Geometry: final body of the model. Coordinates: model frame, mm. A direction names the side the tool comes from. Round coordinates to 2 decimals unless told otherwise and drop trailing zeros. Loops run counter-clockwise (first coordinate to the right, second up) from the corner with the lowest first, then second, coordinate; pieces in that order, holes last. Notation, with made-up numbers: (69.25, 78.5) - (85.25, 78.5) arc R26 cw to (85.25, 114.5) - close; hole circle Ø6 at (-7.75, 65). An arc over 180 degrees is marked (long way). Answer as a JSON object with one key per item and string values. Group by question number.
Item 1: First-contact query: pin 1 (2 mm diameter, centred on x = 21.5, y = 7.5, fed in from -Z); pin 2 (12 mm diameter, centred on y = 9, z = 40.5, fed in from +X) (3 decimals); pin 3 (8 mm diameter, centred on x = 23, y = 17, fed in from +Z); pin 4 (1.5 mm diameter, centred on x = 15.5, z = 23.5, fed in from +Y). Flat tips, straight axial feed; report the tip coordinate or a pass-through.
Item 2: Section C-C (z = 69.5). Return the cut outline in (x, y) (1 decimal), plus the area to 3 significant figures.
Item 3: Reachability of faces 1 (the face through (14, 17.064, 1)), 2 (the face through (4, 12, 1)), 3 (the face through (14.241, 16.004, 31.594)), 4 (the face through (20.63, 9.49, 68.44)), 5 (the face through (20.57, 8.45, 1.48)) from +Z, -Z, +X, -X, +Y, -Y: full face, straight path, thin tool, end or side. Return the list, or none.
Item 4: Line query: line 1 (Z direction, x = 27, y = 25.25); line 2 (Z direction, x = 18.75, y = 10.75); line 3 (Z direction, x = 13, y = 7.25). Output: solid intervals per line, ascending.
Item 5: Section B-B (z = 12.5). Return the cut outline in (x, y) (1 decimal).
Item 6: Section A-A (y = 2.25). Return the cut outline in (x, z).
Item 7: Draft query along Z for faces 6 (the face through (22, 14, 1)), 7 (the face through (14.3, 17.3, 3)). Return one class per face: released by +Z, released by -Z, zero draft, split by the parting line, or undercut.
Autodesk Fusion 360 part; units mm, degrees
sketch "Sketch1" plane through (0, 0, 0) normal (0, 0, 1) x (1, 0, 0)
  line L0 (29, 1.5) -> (29, 26.5)
  line L1 (27.5, 28) -> (1.5, 28)
  line L2 (0, 26.5) -> (0, 1.5)
  line L3 (3, 0) -> (3, 23.5595)
  line L4 (4.5, 25.0595) -> (24.5, 25.0595)
  line L5 (26, 23.5595) -> (26, 4.5)
  line L6 (24.5, 3) -> (8.5, 3)
  line L7 (4, 3) -> (4, 1.5)
  line L8 (4, 3) -> (4, 22.4878)
  line L9 (5.5, 23.9878) -> (23.5, 23.9878)
  line L10 (25, 22.4878) -> (25, 5.5)
  line L11 (23.5, 4) -> (9.5, 4)
  line L12 (8, 5.5) -> (8, 18.4723)
  line L13 (9.5, 19.9723) -> (19.5, 19.9723)
  line L14 (21, 18.4723) -> (21, 9.5)
  line L15 (19.5, 8) -> (13.5173, 8)
  line L16 (12.0173, 9.5) -> (12.0173, 14.3549)
  line L17 (14.0173, 16.3549) -> (15.0961, 16.3549)
  line L18 (17.0961, 14.3549) -> (17.0961, 11)
  line L19 (7, 4.5) -> (7, 19.6029)
  line L20 (8.5, 21.1029) -> (20.5, 21.1029)
  line L21 (22, 19.6029) -> (22, 8.5)
  line L22 (20.5, 7) -> (12.5, 7)
  line L23 (11, 8.5) -> (11, 15.5643)
  line L24 (12.5, 17.0643) -> (16.5, 17.0643)
  line L25 (18, 15.5643) -> (18, 12.3765)
  line L26 (1.5, 0) -> (3, 0)
  line L27 (5.5, 0) -> (27.5, 0)
  circle A0 centre (14.675, 14.0515) radius 2
  arc A1 (1.5, 28) -> (0, 26.5) centre (1.5, 26.5) ccw
  arc A2 (0, 1.5) -> (1.5, 0) centre (1.5, 1.5) ccw
  arc A3 (4.5, 25.0595) -> (3, 23.5595) centre (4.5, 23.5595) ccw
  arc A4 (26, 23.5595) -> (24.5, 25.0595) centre (24.5, 23.5595) ccw
  arc A5 (29, 26.5) -> (27.5, 28) centre (27.5, 26.5) ccw
  arc A6 (27.5, 0) -> (29, 1.5) centre (27.5, 1.5) ccw
  arc A7 (4, 1.5) -> (5.5, 0) centre (5.5, 1.5) ccw
  arc A8 (5.5, 23.9878) -> (4, 22.4878) centre (5.5, 22.4878) ccw
  arc A9 (25, 22.4878) -> (23.5, 23.9878) centre (23.5, 22.4878) ccw
  arc A10 (23.5, 4) -> (25, 5.5) centre (23.5, 5.5) ccw
  arc A11 (24.5, 3) -> (26, 4.5) centre (24.5, 4.5) ccw
  arc A12 (7, 4.5) -> (8.5, 3) centre (8.5, 4.5) ccw
  arc A13 (8, 5.5) -> (9.5, 4) centre (9.5, 5.5) ccw
  arc A14 (9.5, 19.9723) -> (8, 18.4723) centre (9.5, 18.4723) ccw
  arc A15 (8.5, 21.1029) -> (7, 19.6029) centre (8.5, 19.6029) ccw
  arc A16 (22, 19.6029) -> (20.5, 21.1029) centre (20.5, 19.6029) ccw
  arc A17 (21, 18.4723) -> (19.5, 19.9723) centre (19.5, 18.4723) ccw
  arc A18 (20.5, 7) -> (22, 8.5) centre (20.5, 8.5) ccw
  arc A19 (19.5, 8) -> (21, 9.5) centre (19.5, 9.5) ccw
  arc A20 (11, 8.5) -> (12.5, 7) centre (12.5, 8.5) ccw
  arc A21 (12.5, 17.0643) -> (11, 15.5643) centre (12.5, 15.5643) ccw
  arc A22 (18, 15.5643) -> (16.5, 17.0643) centre (16.5, 15.5643) ccw
  arc A23 (17.0961, 11) -> (18, 12.3765) centre (16.5, 12.3765) ccw
  arc A24 (14.0173, 16.3549) -> (12.0173, 14.3549) centre (14.0173, 14.3549) ccw
  arc A25 (17.0961, 14.3549) -> (15.0961, 16.3549) centre (15.0961, 14.3549) ccw
  arc A26 (12.0173, 9.5) -> (13.5173, 8) centre (13.5173, 9.5) ccw
  point P0 (29, 0)
  point P1 (0, 28)
  dimension "d1" = 29
  dimension "d2" = 28
  dimension "d3" = 4
  dimension "d4" = 1.5
  dimension "d5" = 2
  dimension "d15" = 1.5
extrude "Extrude1" add sketch "Sketch1" along normal blind 3
extrude "Extrude2" add sketch "Sketch1" along normal blind 61 contours A0
sketch "Sketch2" plane through (0, 0, 61) normal (0, 0, 1) x (-1, 0, 0)
  circle A0 centre (-14.675, -14.0515) radius 2
  circle A1 centre (-14.675, -14.0515) radius 7.5
  dimension "d10" = 15
extrude "Extrude3" add sketch "Sketch2" along normal blind 15 contours A0 | A1
fillet "Fillet1" radius 3 2 edges at (21.6674, 16.7636, 76) (21.6674, 16.7636, 61)
equation "d8 = 36 mm + 25 mm"
Values:
{
 "1": {"pin 1": "stops at z = 0", "pin 2": "stops at x = 16.675", "pin 3": "stops at z = 75.98", "pin 4": "stops at y = 16.05"},
 "2": {"outline": "circle Ø15 at (14.7, 14.1)", "area": "177 mm^2"},
 "3": {"face 1": "-Z", "face 2": "+Z, -Z, -Y", "face 3": "none", "face 4": "+Z", "face 5": "+Z, -Z"},
 "4": {"line 1": "z = 0 to 3", "line 2": "z = 0 to 3, 61.09 to 75.91", "line 3": "z = 62.35 to 74.65"},
 "5": {"outline": "circle Ø4 at (14.7, 14.1)"},
 "6": {"outline": "(0, 0) - (3, 0) - (3, 3) - (0, 3) - close; (4, 0) - (29, 0) - (29, 3) - (4, 3) - close"},
 "7": {"face 6": "zero draft", "face 7": "undercut"}
}
